Answer from the drawing. Dimensions are ordinates in mm from the lowest x, y and z of the part. Round coordinates to 2 decimals unless told otherwise and drop trailing zeros. Write each loop counter-clockwise with the first axis right and the second up, starting at its lowest first coordinate (ties: lowest second). Pieces come first, ordered by that corner, then holes.
1. Find section A-A (x = 20). Write down the section's boundary in (y, z).
2. Straight lines are drawn through the part: probe 1 along Y at (x, z) = (20, 3.85); probe 2 along Y at (x, z) = (39, 1.95); probe 3 along X at (y, z) = (12.5, 2.65). For each, find the intervals that lie inside material, in ascending order.
3. Find section C-C (y = 13). Write down the section's boundary in (x, z), and give its area (3 significant figures).
4. Find section D-D (z = 1.2). Write down the section's boundary in (x, y), and give its area (3 significant figures).
5. Flat-ended cylindrical pins translate along their axes: pin 1 Ø1.2 at (x, z) = (4, 5) entering from -Y; pin 2 Ø2 at (x, z) = (19.5, 1.5) entering from +Y; pin 3 Ø4 at (x, y) = (39, 13) entering from -Z; pin 4 Ø2 at (y, z) = (3.5, 4.5) entering from -X. Find the tip coordinate at first contact, or state that the pin passes through.
6. Find section B-B (z = 3.9). Write down the section's boundary in (x, y).
7. Determine the mould class of the marked faces 1 and 2 for opening direction X: pulls with the +X half, pulls with the -X half, needs draft (parallel to the pull), parting line crosses it, or undercut.
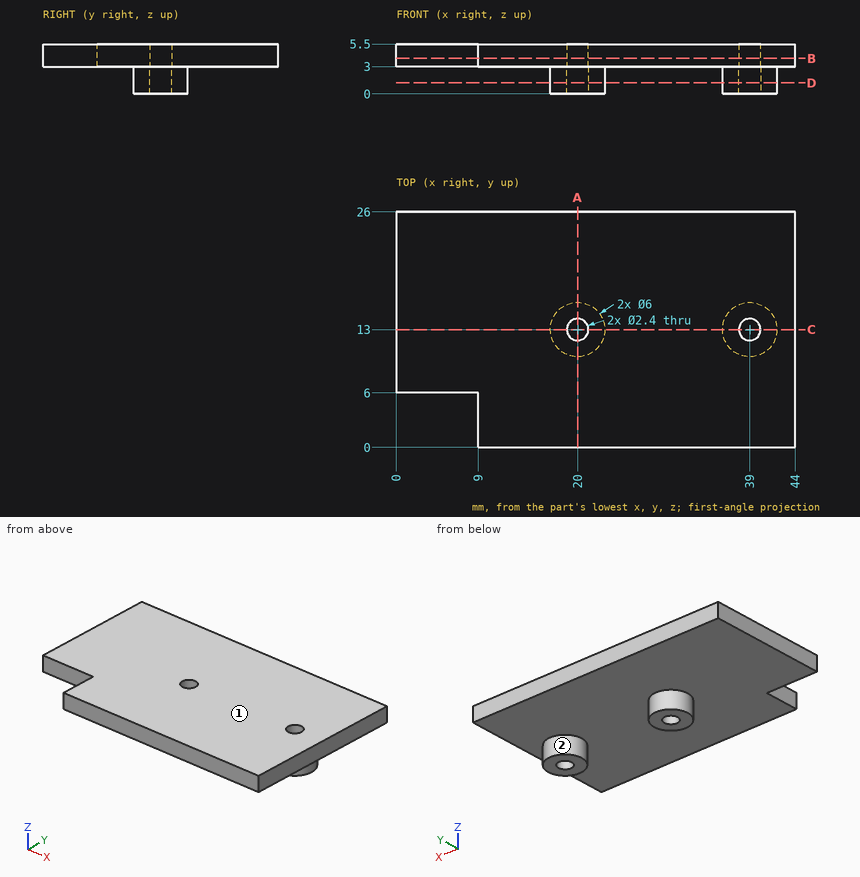
Worked answers:
1. outline: (0, 3) - (10, 3) - (10, 0) - (11.8, 0) - (11.8, 5.5) - (0, 5.5) - close; (14.2, 0) - (16, 0) - (16, 3) - (26, 3) - (26, 5.5) - (14.2, 5.5) - close
2. probe 1: y = 0 to 11.8, 14.2 to 26
2. probe 2: y = 10 to 11.8, 14.2 to 16
2. probe 3: x = 17.04 to 18.91, 21.09 to 22.96, 36.04 to 37.91, 40.09 to 41.96
3. outline: (0, 3) - (17, 3) - (17, 0) - (18.8, 0) - (18.8, 5.5) - (0, 5.5) - close; (21.2, 0) - (23, 0) - (23, 3) - (36, 3) - (36, 0) - (37.8, 0) - (37.8, 5.5) - (21.2, 5.5) - close; (40.2, 0) - (42, 0) - (42, 3) - (44, 3) - (44, 5.5) - (40.2, 5.5) - close
3. area: 120 mm2
4. outline: circle Ø6 at (20, 13); circle Ø6 at (39, 13); hole circle Ø2.4 at (20, 13); hole circle Ø2.4 at (39, 13)
4. area: 47.5 mm2
5. pin 1: stops at y = 6
5. pin 2: stops at y = 16
5. pin 3: stops at z = 0
5. pin 4: stops at x = 9
6. outline: (0, 6) - (9, 6) - (9, 0) - (44, 0) - (44, 26) - (0, 26) - close; hole circle Ø2.4 at (20, 13); hole circle Ø2.4 at (39, 13)
7. face 1: needs draft
7. face 2: undercut
